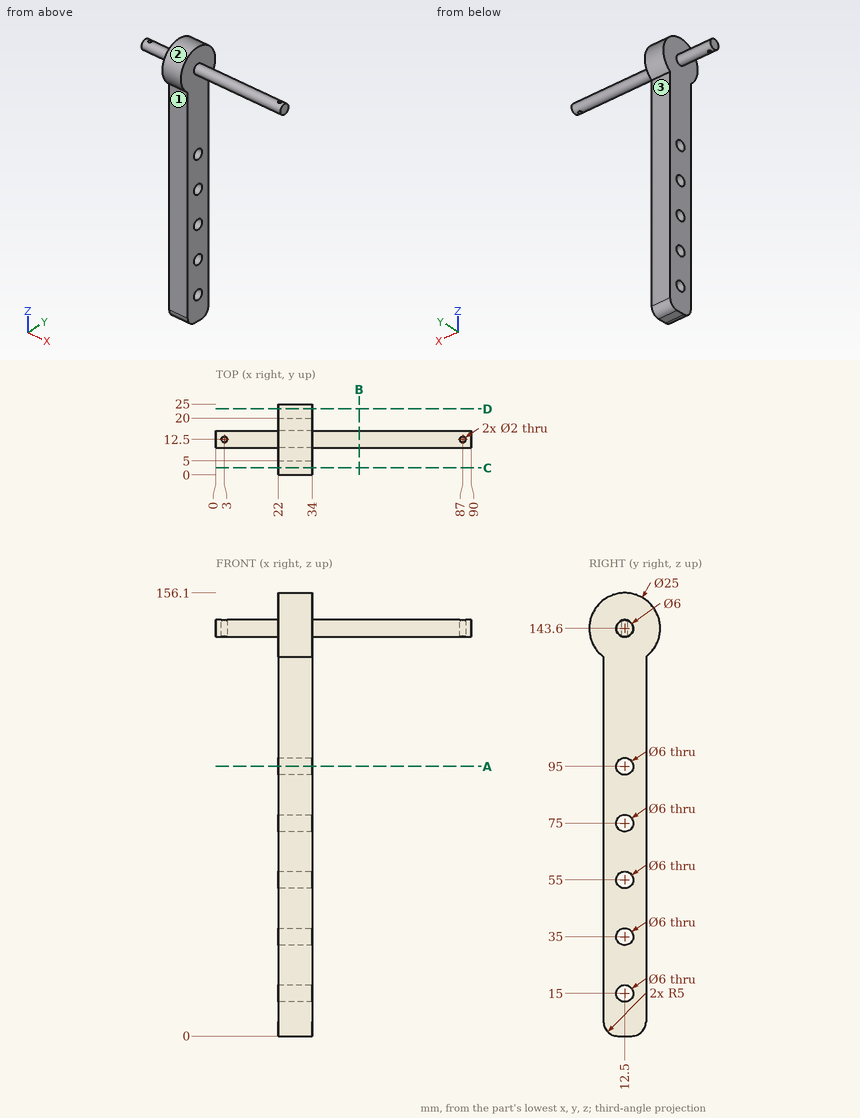
Drawing for the job (mm, zero at the part's lowest x, y, z). A direction names the side the tool comes from. Round coordinates to 2 decimals unless told otherwise and drop trailing zeros. Write each loop counter-clockwise with the first axis right and the second up, starting at its lowest first coordinate (ties: lowest second). Pieces come first, ordered by that corner, then holes. Notation, with made-up numbers: M 76.25,-31.75 L 115.25,-31.75 A17 cw 115.25,-1.75 Z; hole C 71,30.5 d5. An arc over 180 degrees is marked long. Answer in a Markdown table with one row per item.
1. Saw through at C-C (y = 2.5). List the corners of the cut face in (x, z), and give its area (3 significant figures).
Geometry check:
| item | result |
|---|---|
| outline | M 22,136.1 L 34,136.1 L 34,151.1 L 22,151.1 Z |
| area | 180 mm2 |
2. Flat gauge pins, fed straight in: P1, Ø1, axis at y = 18, z = 79.5, coming from the +X side; P2, Ø8, axis at x = 20.5, y = 17, coming from the +Z side; P3, Ø6, axis at x = 28, z = 91.5, coming from the +Y side. Where does each tip first touch, or does it go through?
Geometry check:
| item | result |
|---|---|
| P1 | x = 34 |
| P2 | z = 156.07 |
| P3 | y = 20 |
3. Saw through at D-D (y = 23.25). List the corners of the cut face in (x, z), and give its area (3 significant figures).
Geometry check:
| item | result |
|---|---|
| outline | M 22,137.22 L 34,137.22 L 34,149.98 L 22,149.98 Z |
| area | 153 mm2 |
4. Saw through at B-B (x = 50.5). List the corners of the cut face in (y, z).
Geometry check:
| item | result |
|---|---|
| outline | C 12.5,143.6 d6 |
5. Probe L1, parallel to Z at x = 32, y = 12.25; L2, parallel to X at y = 12.5, z = 142.25; L3, parallel to X at y = 19.75, z = 90. List the from-to ranges inside material, lowest first. Write a range as [from, to].
Geometry check:
| item | result |
|---|---|
| L1 | [0, 12.01], [17.99, 32.01], [37.99, 52.01], [57.99, 72.01], [77.99, 92.01], [97.99, 156.1] |
| L2 | [0, 2], [4, 86], [88, 90] |
| L3 | [22, 34] |
6. Saw through at A-A (z = 95). List the corners of the cut face in (x, y), and give its area (3 significant figures).
Geometry check:
| item | result |
|---|---|
| outline | M 22,5 L 34,5 L 34,9.5 L 22,9.5 Z; M 22,15.5 L 34,15.5 L 34,20 L 22,20 Z |
| area | 108 mm2 |
7. Which spindle directions (+Z, -Z, +X, -X, +Y, -Y) get a long thin tool onto all of the face, cutting with end or side? Do the marked faces 1, 2 and 3. Say none if no direction does.
Geometry check:
| item | result |
|---|---|
| face 1 | -Z, +X, -X, -Y |
| face 2 | +X, -X |
| face 3 | -Z, +X, -X, +Y |
